```python
from build123d import *

# Parameters (mm, degrees)
BOSS_EXTRUDE1_DEPTH = 28
BOSS_EXTRUDE2_DEPTH = 2
CUT_EXTRUDE1_DEPTH  = 20.25


with BuildPart() as part:
    # Sketch1 → Boss-Extrude1 (new body)
    with BuildSketch(Plane.XY):
        with BuildLine():
            ThreePointArc((-17.05, 16.75), (-16.317766953, 18.517766953), (-14.55, 19.25))
            Line((-14.55, 19.25), (14.55, 19.25))
            ThreePointArc((14.55, 19.25), (16.317766953, 18.517766953), (17.05, 16.75))
            Line((17.05, 16.75), (17.05, -16.75))
            ThreePointArc((17.05, -16.75), (16.317766953, -18.517766953), (14.55, -19.25))
            Line((14.55, -19.25), (-14.55, -19.25))
            ThreePointArc((-14.55, -19.25), (-16.317766953, -18.517766953), (-17.05, -16.75))
            Line((-17.05, -16.75), (-17.05, 16.75))
        make_face()
        with BuildLine():
            Line((-14.55, -18.4), (14.55, -18.4))
            ThreePointArc((14.55, -18.4), (15.716726189, -17.916726189), (16.2, -16.75))
            Line((16.2, -16.75), (16.2, 16.75))
            ThreePointArc((16.2, 16.75), (15.716726189, 17.916726189), (14.55, 18.4))
            Line((14.55, 18.4), (-14.55, 18.4))
            ThreePointArc((-14.55, 18.4), (-15.716726189, 17.916726189), (-16.2, 16.75))
            Line((-16.2, 16.75), (-16.2, -16.75))
            ThreePointArc((-16.2, -16.75), (-15.716726189, -17.916726189), (-14.55, -18.4))
        make_face(mode=Mode.SUBTRACT)
    extrude(amount=BOSS_EXTRUDE1_DEPTH)

    # Sketch1_3 → Boss-Extrude2 (add)
    with BuildSketch(Plane.XY):
        with BuildLine():
            ThreePointArc((-14.55, -18.4), (-15.716726189, -17.916726189), (-16.2, -16.75))
            Line((-16.2, -16.75), (-16.2, 16.75))
            ThreePointArc((-16.2, 16.75), (-15.716726189, 17.916726189), (-14.55, 18.4))
            Line((-14.55, 18.4), (14.55, 18.4))
            ThreePointArc((14.55, 18.4), (15.716726189, 17.916726189), (16.2, 16.75))
            Line((16.2, 16.75), (16.2, -16.75))
            ThreePointArc((16.2, -16.75), (15.716726189, -17.916726189), (14.55, -18.4))
            Line((14.55, -18.4), (-14.55, -18.4))
        make_face()
        with BuildLine():
            Line((-10, -15.4), (-10, -9.4))
            ThreePointArc((-10, -9.4), (-9.707106781, -8.692893219), (-9, -8.4))
            Line((-9, -8.4), (9, -8.4))
            ThreePointArc((9, -8.4), (9.707106781, -8.692893219), (10, -9.4))
            Line((10, -9.4), (10, -15.4))
            ThreePointArc((10, -15.4), (9.707106781, -16.107106781), (9, -16.4))
            Line((9, -16.4), (-9, -16.4))
            ThreePointArc((-9, -16.4), (-9.707106781, -16.107106781), (-10, -15.4))
        make_face(mode=Mode.SUBTRACT)
    extrude(amount=BOSS_EXTRUDE2_DEPTH)

    # Sketch2 → Cut-Extrude1 (cut, through all)
    with BuildSketch(Plane(origin=(0, 0, 0), x_dir=(1, 0, 0), z_dir=(0, 1, 0))):
        with BuildLine():
            Line((-12, -28), (12, -28))
            Line((12, -28), (12, -22))
            ThreePointArc((12, -22), (11.707106781, -21.292893219), (11, -21))
            Line((11, -21), (-11, -21))
            ThreePointArc((-11, -21), (-11.707106781, -21.292893219), (-12, -22))
            Line((-12, -22), (-12, -28))
        make_face()
    extrude(amount=CUT_EXTRUDE1_DEPTH, mode=Mode.SUBTRACT)


solid = part.part
```
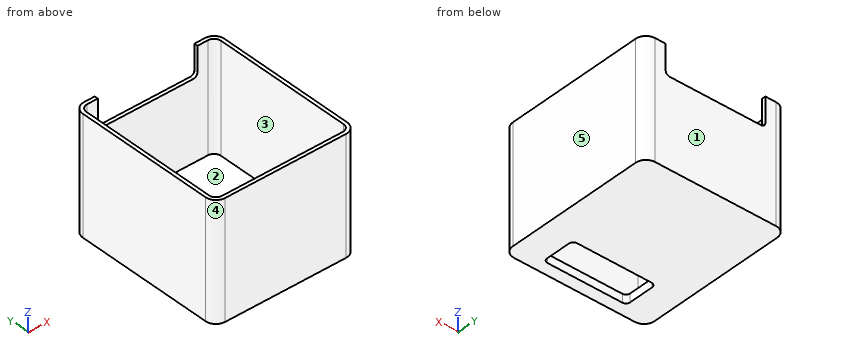
CAD build for the part. Positions are in the model's coordinates, mm. Face numbers are marked on the shaded views. A direction names the side the tool comes from. Coordinates: 2 decimals unless noted, no trailing zeros. Order: outer loops, then holes, each group sorted by start corner. A loop starts at its lowest first (then second) coordinate and runs counter-clockwise, first axis right, second up. Notation, with made-up numbers: (57.25, -34) - (114.25, -34) arc R32 cw to (114.25, 2) - close; hole circle Ø11 at (21.5, -28.75). An arc over 180 degrees is marked (long way). Use a Markdown table: item, result. Add a question column.
(1) Saw through at B-B (z = 24). Give the cut face in (x, y).
(2) Which spindle directions (+Z, -Z, +X, -X, +Y, -Y) get a long thin tool onto all of the face, cutting with end or side? Do the marked faces 1 and 2. Say none if no direction does.
(3) Drill centre lines: line 1 along Y through (x, z) = (-4, 5.75); line 2 along X through (y, z) = (-3.5, 16); line 3 along X through (y, z) = (-12.5, 1.5). Where is each one in solid material? Low to high. Write a range as [from, to].
(4) Saw through at C-C (y = -10). Give the cut face in (x, z), then the cut area to 3 significant figures.
(5) Saw through at D-D (z = 10). Give the cut face in (x, y), then the cut area to 3 significant figures.
(6) Flat gauge pins, fed straight in: pin 1 (6 mm diameter, centred on x = 7.5, y = 0, fed in from +Z); pin 2 (0.7 mm diameter, centred on y = 18.5, z = 25, fed in from -X). Where does each tip first touch, or does it go through?
(7) Pull direction X, two halves, no side cores. Call the marked faces 3, 4 and 5: +X half, -X half, draft (parallel to the pull), parting line (faces both ways), or undercut.
(8) Saw through at A-A (x = 3.5). Give the cut face in (y, z).
Solved:
| question | item | result |
|---|---|---|
| 1 | outline | (-17.05, -16.75) arc R2.5 ccw to (-14.55, -19.25) - (14.55, -19.25) arc R2.5 ccw to (17.05, -16.75) - (17.05, 16.75) arc R2.5 ccw to (14.55, 19.25) - (12, 19.25) - (12, 18.4) - (14.55, 18.4) arc R1.65 cw to (16.2, 16.75) - (16.2, -16.75) arc R1.65 cw to (14.55, -18.4) - (-14.55, -18.4) arc R1.65 cw to (-16.2, -16.75) - (-16.2, 16.75) arc R1.65 cw to (-14.55, 18.4) - (-12, 18.4) - (-12, 19.25) - (-14.55, 19.25) arc R2.5 ccw to (-17.05, 16.75) - close |
| 2 | face 1 | +Z, -Z, +X, -X, +Y |
| 2 | face 2 | +Z |
| 3 | line 1 | y = [-19.25, -18.4], [18.4, 19.25] |
| 3 | line 2 | x = [-17.05, -16.2], [16.2, 17.05] |
| 3 | line 3 | x = [-17.05, -10], [10, 17.05] |
| 4 | outline | (-17.05, 0) - (-10, 0) - (-10, 2) - (-16.2, 2) - (-16.2, 28) - (-17.05, 28) - close; (10, 0) - (17.05, 0) - (17.05, 28) - (16.2, 28) - (16.2, 2) - (10, 2) - close |
| 4 | area | 72.4 mm² |
| 5 | outline | (-17.05, -16.75) arc R2.5 ccw to (-14.55, -19.25) - (14.55, -19.25) arc R2.5 ccw to (17.05, -16.75) - (17.05, 16.75) arc R2.5 ccw to (14.55, 19.25) - (-14.55, 19.25) arc R2.5 ccw to (-17.05, 16.75) - close; hole (-16.2, -16.75) arc R1.65 ccw to (-14.55, -18.4) - (14.55, -18.4) arc R1.65 ccw to (16.2, -16.75) - (16.2, 16.75) arc R1.65 ccw to (14.55, 18.4) - (-14.55, 18.4) arc R1.65 ccw to (-16.2, 16.75) - close |
| 5 | area | 118 mm² |
| 6 | pin 1 | stops at z = 2 |
| 6 | pin 2 | stops at x = -16.62 |
| 7 | face 3 | undercut |
| 7 | face 4 | -X half |
| 7 | face 5 | +X half |
| 8 | outline | (-19.25, 0) - (-16.4, 0) - (-16.4, 2) - (-18.4, 2) - (-18.4, 28) - (-19.25, 28) - close; (-8.4, 0) - (19.25, 0) - (19.25, 21) - (18.4, 21) - (18.4, 2) - (-8.4, 2) - close |
